The model under review builds one solid part; all positions refer to its coordinate system, in mm. A direction names the side the tool comes from. Coordinates: 2 decimals unless noted, no trailing zeros. Order: outer loops, then holes, each group sorted by start corner. A loop starts at its lowest first (then second) coordinate and runs counter-clockwise, first axis right, second up. Notation, with made-up numbers: M -2,88 L 46,88 A21 cw 46,100 Z; hole C 9,-13 d8. An arc over 180 degrees is marked long. One line per item, written item: value.
```python
from build123d import *

# Parameters (mm, degrees)
F0_W     = 180
F0_H     = 30
F0_W_2   = 110
F0_H_2   = 16
F1_DEPTH = 5
F2_R     = 11
F2_R_2   = 0.5
F2_R_3   = 2.75
F2_W     = 24.5
F2_H     = 12
F3_DEPTH = 3
F2_R_4   = 0.75
F4_DEPTH = 25
F5_R     = 14.99999
F6_R     = 7
F7_R     = 0.5


# Not quite as in the source:
# - a fillet or chamfer is up to 0.001 mm smaller than in the source, because OpenCascade refuses the exact size
# - a feature names something its author has since deleted; it is built from what else it names


with BuildPart() as f1:
    # F0 (on Top) → F1 (new body)
    with BuildSketch(Plane.XY):
        with Locations((10, -11.8972941886)):
            Rectangle(F0_W, F0_H)
        with Locations((15, -11.8972941886)):
            Rectangle(F0_W_2, F0_H_2, mode=Mode.SUBTRACT)
    extrude(amount=F1_DEPTH)

    # F2 (on face) → F3 (cut)
    with BuildSketch(Plane.XY.offset(5)):
        with Locations((85, -11.8972941886)):
            Circle(F2_R)
        with Locations((85, -18.8972941886)):
            Circle(F2_R_2, mode=Mode.SUBTRACT)
        with Locations((85, -11.8972941886)):
            Circle(F2_R_3, mode=Mode.SUBTRACT)
        with Locations((78, -11.8972941886)):
            Circle(F2_R_2, mode=Mode.SUBTRACT)
        with Locations((92, -11.8972941886)):
            Circle(F2_R_2, mode=Mode.SUBTRACT)
        with Locations((85, -4.8972941886)):
            Circle(F2_R_2, mode=Mode.SUBTRACT)
        with Locations((-60.75, -11.8972941886)):
            Rectangle(F2_W, F2_H)
        with Locations((-65, -11.8972941886)):
            Circle(F2_R_3, mode=Mode.SUBTRACT)
    extrude(amount=-F3_DEPTH, mode=Mode.SUBTRACT)

    # F2 (on face) → F4 (cut)
    with BuildSketch(Plane.XY.offset(5)):
        with Locations((-60.75, -11.8972941886)):
            Rectangle(F2_W, F2_H)
        with Locations((-65, -11.8972941886)):
            Circle(F2_R_3, mode=Mode.SUBTRACT)
        with Locations((85, -11.8972941886)):
            Circle(F2_R_3)
        with Locations((-65, -11.8972941886)):
            Circle(F2_R_3)
        with Locations((-76, -11.8972941886)):
            Circle(F2_R_4)
        with Locations((-45.5, -11.8972941886)):
            Circle(F2_R_4)
        with Locations((85, -4.8972941886)):
            Circle(F2_R_2)
        with Locations((78, -11.8972941886)):
            Circle(F2_R_2)
        with Locations((85, -18.8972941886)):
            Circle(F2_R_2)
        with Locations((92, -11.8972941886)):
            Circle(F2_R_2)
    extrude(amount=-F4_DEPTH, mode=Mode.SUBTRACT)

    # F5 (radius 15 in the source; OpenCascade refuses exactly that, so slightly less here)
    f5_edges = [f1.edges().sort_by_distance(p)[0] for p in [
        (100, 3.102706, 2.5),
        (100, -26.897294, 2.5),
        (-80, -26.897294, 2.5),
        (-80, 3.102706, 2.5),
    ]]
    fillet(f5_edges, radius=F5_R)

    # F6
    f6_edges = [f1.edges().sort_by_distance(p)[0] for p in [
        (-40, -3.897294, 2.5),
        (-40, -19.897294, 2.5),
        (70, -3.897294, 2.5),
        (70, -19.897294, 2.5),
    ]]
    fillet(f6_edges, radius=F6_R)

    # F7
    f7_edges = [f1.edges().sort_by_distance(p)[0] for p in [
        (-73, -5.897294, 2.5),
        (-73, -17.897294, 2.5),
        (-48.5, -5.897294, 2.5),
        (-48.5, -17.897294, 2.5),
    ]]
    fillet(f7_edges, radius=F7_R)


solid = f1.part
```
(1) We need section B-B, the plane z = 3.75. Count the separate pieces of the cut face and the enclosed holes in it, plus the area to 3 significant figures.
Geometry results:
separate pieces: 1
enclosed holes: 5
area: 2,810 mm2
(2) We need section A-A, the plane x = 58.5. State the section outline as (y, z) points, plus the area to 3 significant figures.
Geometry results:
outline: M -26.9,0 L -19.9,0 L -19.9,5 L -26.9,5 Z; M -3.9,0 L 3.1,0 L 3.1,5 L -3.9,5 Z
area: 70.0 mm2
(3) For L1, parallel to Y at x = 42.5, z = 2.75; L2, parallel to X at y = -11, z = 4.6; L3, parallel to X at y = -11.5, z = 2.35, list the stretches that pass through material, from the lowest coordinate up.
Geometry results:
L1: y = -26.9 to -19.9, -3.9 to 3.1
L2: x = -79.97 to -73, -48.5 to -40, 70 to 74.04, 95.96 to 99.97
L3: x = -79.99 to -76.64, -75.36 to -73, -48.5 to -46.14, -44.86 to -40, 70 to 74.01, 95.99 to 99.99
(4) Mouldability with a two-part tool opening along X and no side actions: class faces 4 (the cylindrical face through (67.895, -17.901, 2.535)), 5 (the cylindrical face through (-75.723, -1.408, 2.535)), 6 (the flat face through (9, -26.897, 2)) as +X half, -X half, draft (parallel to the pull), parting line (faces both ways), or undercut.
Geometry results:
face 4: undercut
face 5: -X half
face 6: draft
(5) We need section C-C, the plane x = -53. State the section outline as (y, z) points.
Geometry results:
outline: M -26.9,0 L -17.9,0 L -17.9,5 L -26.9,5 Z; M -5.9,0 L 3.1,0 L 3.1,5 L -5.9,5 Z
(6) We need section D-D, the plane y = 1. State the section outline as (x, z) points.
Geometry results:
outline: M -72.66,0 L 92.66,0 L 92.66,5 L -72.66,5 Z
(7) Insertion check: pin 1 Ø5 at (x, y) = (13, -18.5) entering from -Z; pin 2 Ø1.5 at (y, z) = (-14.5, 3) entering from -X; pin 3 Ø6.5 at (x, y) = (89.5, -8.5) entering from +Z. Each pin has a flat end and moves straight along its axis. Give the tip position at first contact, or say it passes through.
Geometry results:
pin 1: stops at z = 0
pin 2: stops at x = -79.89
pin 3: stops at z = 2
(8) Tool access review of faces 1 (the flat face through (9, -2, 5)), 2 (the flat face through (-61, -17.897, 3)), 3 (the flat face through (87, -14, 2)): name each direction out of +Z, -Z, +X, -X, +Y, -Y from which nothing blocks a thin tool from reaching the whole face with its end or side.
Geometry results:
face 1: +Z, +X, -X, +Y, -Y
face 2: +Z, -Z
face 3: +Z
